Here's the drawing with two shaded views (mm, measured from the low corner). I have some questions. A direction names the side the tool comes from. Coordinates: 2 decimals unless noted, no trailing zeros. Loops run counter-clockwise (first coordinate to the right, second up) from the corner with the lowest first, then second, coordinate; pieces in that order, holes last. Notation, with made-up numbers: (69, 63) -> (86, 63) arc R21 ccw to (86, 95) -> close; hole circle Ø6 at (-7.5, 18.25). An arc over 180 degrees is marked (long way). Answer as a JSON object with one key per item and string values. Group by question number.
1) I need wall thicknesses on probe 1 along X at (y, z) = (1.5, 11.5); probe 2 along Y at (x, z) = (23, 8); probe 3 along X at (y, z) = (3.9, 2.25). Which ranges of each line are inside material? Lowest first, please. Write a range as [from, to].
2) I'm going to push flat-ended pins straight in: pin 1 (1.3 mm diameter, centred on y = 2, z = 13.5, fed in from -X); pin 2 (1.5 mm diameter, centred on x = 8.5, z = 3.5, fed in from -Y); pin 3 (4 mm diameter, centred on x = 20.5, z = 7, fed in from +Y). Where does each tip first touch, or does it pass through?
3) I want a section at D-D (z = 12). Write out the boundary of the cut face in (x, y).
4) I want a section at A-A (y = 3.05). Write out the boundary of the cut face in (x, z) (1 decimal), then the cut area to 3 significant figures.
5) If we mould it in two halves opening along Y, with no side actions, what happens to the marked faces 1, 2 and 3? For each: +Y half, -Y half, draft (parallel to the pull), parting line (faces both ways), or undercut.
6) Which directions (+Z, -Z, +X, -X, +Y, -Y) give clear straight access to the entire face, cutting with the end or side of a thin tool? Please do the marked faces 4, 5 and 6.
7) I want a section at C-C (x = 6.25). Write out the boundary of the cut face in (y, z).
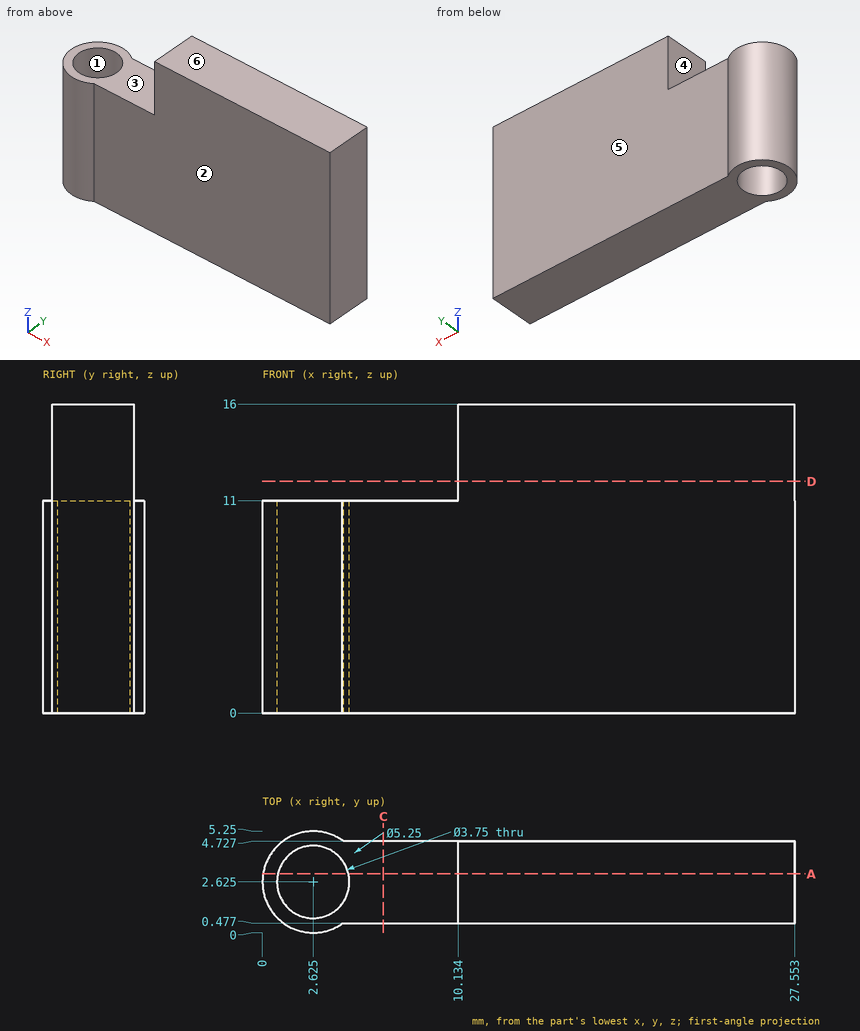
Determined:
{
 "1": {"probe 1": "[10.13, 27.55]", "probe 2": "[0.48, 4.73]", "probe 3": "[0.33, 1.25], [4, 27.55]"},
 "2": {"pin 1": "x = 10.13", "pin 2": "y = 0.48", "pin 3": "y = 4.73"},
 "3": {"outline": "(10.13, 0.48) -> (27.55, 0.48) -> (27.55, 4.73) -> (10.13, 4.73) -> close"},
 "4": {"outline": "(0, 0) -> (0.8, 0) -> (0.8, 11) -> (0, 11) -> close; (4.5, 0) -> (27.6, 0) -> (27.6, 16) -> (10.1, 16) -> (10.1, 11) -> (4.5, 11) -> close", "area": "350 mm^2"},
 "5": {"face 1": "undercut", "face 2": "-Y half", "face 3": "draft"},
 "6": {"face 4": "+Z, -X, +Y, -Y", "face 5": "+Z, -Z, +X, +Y", "face 6": "+Z, +X, -X, +Y, -Y"},
 "7": {"outline": "(0.48, 0) -> (4.73, 0) -> (4.73, 11) -> (0.48, 11) -> close"}
}
